```python
from build123d import *

# Parameters (mm, degrees)
SKETCH1_W                        = 209.55
SKETCH1_H                        = 279.399995444
SKETCH1_R                        = 2.5273
BOSS_EXTRUDE1_DEPTH              = 3.175
SKETCH2_W                        = 222.25
SKETCH2_H                        = 292.099995444
SKETCH2_W_2                      = 212.725
SKETCH2_H_2                      = 282.574995444
BOSS_EXTRUDE2_DEPTH              = 12.7
SKETCH2_2_W                      = 212.725
SKETCH2_2_H                      = 282.574995444
SKETCH2_2_W_2                    = 209.55
SKETCH2_2_H_2                    = 279.399995444
BOSS_EXTRUDE3_DEPTH              = 3.175
F_39_64_0_60938_DIAMETER_HOLE1_D = 15.478252


with BuildPart() as part:
    # Sketch1 → Boss-Extrude1 (new body)
    with BuildSketch(Plane(origin=(0, 0, 0), x_dir=(1, 0, 0), z_dir=(0, 1, 0))):
        with Locations((-68.646181354, 29.300553278)):
            Rectangle(SKETCH1_W, SKETCH1_H)
        with Locations((-167.421181354, -104.399444444)):
            Circle(SKETCH1_R, mode=Mode.SUBTRACT)
        with Locations((-167.421181354, 163.000555634)):
            Circle(SKETCH1_R, mode=Mode.SUBTRACT)
        with Locations((30.128818646, -104.399444444)):
            Circle(SKETCH1_R, mode=Mode.SUBTRACT)
        with Locations((30.128818646, 163.000555634)):
            Circle(SKETCH1_R, mode=Mode.SUBTRACT)
    extrude(amount=BOSS_EXTRUDE1_DEPTH)



with BuildPart() as body_2:
    # Sketch2 → Boss-Extrude2 (new body)
    with BuildSketch(Plane(origin=(0, 3.175, 0), x_dir=(1, 0, 0), z_dir=(0, 1, 0))):
        with Locations((-68.646181354, 29.300553278)):
            Rectangle(SKETCH2_W, SKETCH2_H)
        with Locations((-68.646181354, 29.300553278)):
            Rectangle(SKETCH2_W_2, SKETCH2_H_2, mode=Mode.SUBTRACT)
    extrude(amount=-BOSS_EXTRUDE2_DEPTH)


with BuildPart() as part_1:
    add(part.part)

    add(body_2.part)  # Boss-Extrude3 merges body 2
    # Sketch2<2> → Boss-Extrude3 (add)
    with BuildSketch(Plane(origin=(0, 3.175, 0), x_dir=(1, 0, 0), z_dir=(0, 1, 0))):
        with Locations((-68.646181354, 29.300553278)):
            Rectangle(SKETCH2_2_W, SKETCH2_2_H)
        with Locations((-68.646181354, 29.300553278)):
            Rectangle(SKETCH2_2_W_2, SKETCH2_2_H_2, mode=Mode.SUBTRACT)
    extrude(amount=-BOSS_EXTRUDE3_DEPTH)

    # 39/64 (0.60938) Diameter Hole1 (through all)
    with Locations(Plane(origin=(0, 3.175, 0), x_dir=(1, 0, 0), z_dir=(0, 1, 0))):
        with Locations((-69.646181393, 110.086655576), (-48.646181397, 107.086655551), (-69.64618139, 87.226655576), (-48.646181393, 84.226655551), (-48.64618139, 61.366655551), (-69.646181387, 64.366655576), (-69.646181383, 41.506655576), (-48.646181387, 38.506655551), (-48.646181384, 15.646655551), (-69.64618138, 18.646655576), (-69.646181377, -4.213344424), (-48.646181381, -7.213344449), (-48.646181377, -30.073344449), (-69.646181374, -27.073344424), (-69.646181371, -49.933344424), (-48.646181374, -52.933344449)):
            Hole(F_39_64_0_60938_DIAMETER_HOLE1_D / 2)


solid = part_1.part
```
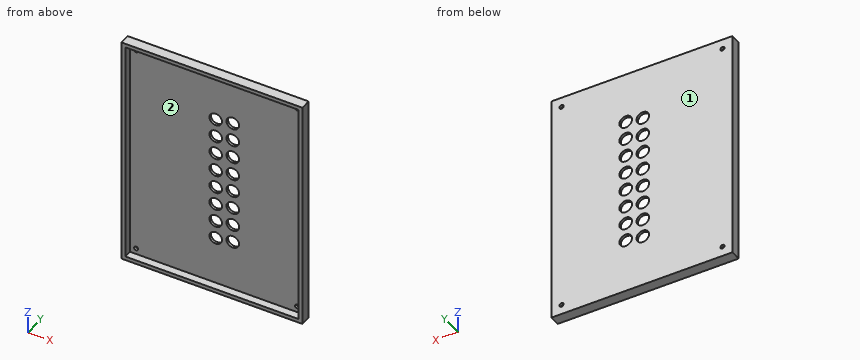
Design review of the part built by this model. Coordinates are the model's own, in mm. Face numbers are marked on the shaded views. Round coordinates to 2 decimals unless told otherwise and drop trailing zeros. Write each loop counter-clockwise with the first axis right and the second up, starting at its lowest first coordinate (ties: lowest second). Pieces come first, ordered by that corner, then holes.
Item 1: We need section B-B on x = -85.5. Write out the cut boundary in (y, z) (3 decimals).
Item 2: Clearance check with a flat-ended pin moving along its axis: pin 1 Ø6 at (x, z) = (30.13, -163) entering from -Y. State where the tip first meets the part, or that it passes through.
Item 3: We need section A-A on y = -6.25. Write out the cut boundary in (x, z).
Item 4: We need section C-C on z = -140.5. Write out the cut boundary in (x, y) (3 decimals), and give its area (3 significant figures).
Item 5: The part is to be moulded in two halves that separate along Z. For the marked faces 1 and 2, say which applies: +Z half, -Z half, draft (parallel to the pull), parting line (faces both ways), or undercut.
Item 6: For probe 1 along Z at (x, y) = (30, 0.5); probe 2 along Z at (x, y) = (-18.5, -8); probe 3 along X at (y, z) = (-4.5, -44.5), list the stretches that pass through material, from the lowest coordinate up.
Returned:
1. outline: (-9.525, -175.351) - (3.175, -175.351) - (3.175, 116.749) - (-9.525, 116.749) - (-9.525, 111.987) - (0, 111.987) - (0, -170.588) - (-9.525, -170.588) - close
2. pin 1: stops at y = 0
3. outline: (-179.77, -175.35) - (42.48, -175.35) - (42.48, 116.75) - (-179.77, 116.75) - close; hole (-175.01, -170.59) - (37.72, -170.59) - (37.72, 111.99) - (-175.01, 111.99) - close
4. outline: (-179.771, -9.525) - (-175.009, -9.525) - (-175.009, 0) - (37.716, 0) - (37.716, -9.525) - (42.479, -9.525) - (42.479, 3.175) - (-179.771, 3.175) - close
4. area: 796 mm2
5. face 1: draft
5. face 2: undercut
6. probe 1: z = -175.35 to -165.52, -160.48 to 101.88, 106.92 to 116.75
6. probe 2: z = -175.35 to -170.59, 111.99 to 116.75
6. probe 3: x = -179.77 to -175.01, 37.72 to 42.48
